```python
from build123d import *

# Parameters (mm, degrees)
SKETCH2_W               = 90
SKETCH2_H               = 45
BOSS_EXTRUDE1_DEPTH     = 8
SKETCH3_R               = 3.25
CUT_EXTRUDE1_DEPTH      = 10
SKETCH5_R               = 5.5
CUT_EXTRUDE2_DEPTH      = 5
SKETCH6_W               = 90
SKETCH6_H               = 5
BOSS_EXTRUDE2_DEPTH     = 32.5
SKETCH7_W               = 90
SKETCH7_H               = 3
BOSS_EXTRUDE3_DEPTH     = 45
SKETCH8_R               = 13
CUT_EXTRUDE4_DEPTH      = 13
BOSS_EXTRUDE6_START     = 5
SKETCH11_R              = 15
SKETCH11_R_2            = 13
BOSS_EXTRUDE6_DEPTH     = 5
FILLET1_R               = 2
CUT_EXTRUDE5_START      = -2
SKETCH12_R              = 13
CUT_EXTRUDE5_DEPTH      = 2
CUT_EXTRUDE6_DEPTH      = 67.494360663
CUT_EXTRUDE6_DEPTH_BACK = 67.494360663
SKETCH13_R              = 3
SKETCH14_R              = 9
CUT_EXTRUDE7_DEPTH      = 12
SKETCH16_W              = 90
SKETCH16_H              = 8
BOSS_EXTRUDE7_DEPTH     = 5
FILLET2_R               = 5


with BuildPart() as part:
    # Sketch2 → Boss-Extrude1 (new body)
    with BuildSketch(Plane(origin=(0, 0, 0), x_dir=(1, 0, 0), z_dir=(0, 1, 0))):
        Rectangle(SKETCH2_W, SKETCH2_H)
    extrude(amount=BOSS_EXTRUDE1_DEPTH)

    # Sketch3 → Cut-Extrude1 (cut)
    with BuildSketch(Plane(origin=(0, 8, 0), x_dir=(1, 0, 0), z_dir=(0, 1, 0))):
        with Locations(Location((12.5, 0, 0), (0, 0, 270))):
            Circle(SKETCH3_R)
        with Locations(Location((-12.5, 0, 0), (0, 0, 270))):
            Circle(SKETCH3_R)
    extrude(amount=-CUT_EXTRUDE1_DEPTH, mode=Mode.SUBTRACT)

    # Sketch5 → Cut-Extrude2 (cut)
    with BuildSketch(Plane(origin=(0, 8, 0), x_dir=(1, 0, 0), z_dir=(0, 1, 0))):
        with Locations(Location((-12.5, 0, 0), (0, 0, 270))):
            Circle(SKETCH5_R)
        with Locations(Location((12.5, 0, 0), (0, 0, 270))):
            Circle(SKETCH5_R)
    extrude(amount=-CUT_EXTRUDE2_DEPTH, mode=Mode.SUBTRACT)

    # Sketch6 → Boss-Extrude2 (add)
    with BuildSketch(Plane(origin=(0, 8, 0), x_dir=(1, 0, 0), z_dir=(0, 1, 0))):
        with Locations((0, -20)):
            Rectangle(SKETCH6_W, SKETCH6_H)
    extrude(amount=BOSS_EXTRUDE2_DEPTH)

    # Sketch7 → Boss-Extrude3 (add)
    with BuildSketch(Plane(origin=(0, 0, 17.5), x_dir=(-1, 0, 0), z_dir=(0, 0, -1))):
        with Locations((0, 39)):
            Rectangle(SKETCH7_W, SKETCH7_H)
    extrude(amount=BOSS_EXTRUDE3_DEPTH)

    # Sketch8 → Cut-Extrude4 (cut)
    with BuildSketch(Plane.XY.offset(22.5)):
        with Locations((0.439882225, 22.012295082)):
            Circle(SKETCH8_R)
    extrude(amount=-CUT_EXTRUDE4_DEPTH, mode=Mode.SUBTRACT)

    # Sketch11 → Boss-Extrude6 (add)
    with BuildSketch(Plane.XY.offset(22.5).offset(BOSS_EXTRUDE6_START)):
        with Locations(Location((0.439882225, 22.012295082, 0), (0, 0, 180))):
            Circle(SKETCH11_R)
        with Locations((0.439882225, 22.012295082)):
            Circle(SKETCH11_R_2, mode=Mode.SUBTRACT)
    extrude(amount=-BOSS_EXTRUDE6_DEPTH)

    # Fillet1
    fillet1_edges = [part.edges().sort_by_distance(p)[0] for p in [
        (15.439882225, 22.012295082, 22.5),
    ]]
    fillet(fillet1_edges, radius=FILLET1_R)

    # Sketch12 → Cut-Extrude5 (cut)
    with BuildSketch(Plane(origin=(0, 0, 17.5), x_dir=(-1, 0, 0), z_dir=(0, 0, -1)).offset(CUT_EXTRUDE5_START)):
        with BuildLine():
            Line((-28.100883588, 8), (27.221119137, 8))
            ThreePointArc((27.221119137, 8), (30.795754245, 22.781960072), (26.966438327, 37.5))
            Line((26.966438327, 37.5), (-27.846202777, 37.5))
            ThreePointArc((-27.846202777, 37.5), (-31.675518695, 22.781960072), (-28.100883588, 8))
        make_face()
        with Locations(Location((-0.439882225, 22.012295082, 0), (0, 0, 180))):
            Circle(SKETCH12_R, mode=Mode.SUBTRACT)
    extrude(amount=CUT_EXTRUDE5_DEPTH, mode=Mode.SUBTRACT)

    # Sketch13 → Cut-Extrude6 (cut, two sides: drawn at the far end of the back side and taken through both)
    with BuildSketch(Plane(origin=(0, 40.5, 0), x_dir=(1, 0, 0), z_dir=(0, 1, 0)).offset(-CUT_EXTRUDE6_DEPTH_BACK)):
        with Locations(Location((-30, 17.5, 0), (0, 0, 270))):
            Circle(SKETCH13_R)
        with Locations(Location((-10, 17.5, 0), (0, 0, 270))):
            Circle(SKETCH13_R)
        with Locations(Location((10, 17.5, 0), (0, 0, 270))):
            Circle(SKETCH13_R)
        with Locations(Location((30, 17.5, 0), (0, 0, 270))):
            Circle(SKETCH13_R)
    extrude(amount=CUT_EXTRUDE6_DEPTH + CUT_EXTRUDE6_DEPTH_BACK, mode=Mode.SUBTRACT)

    # Sketch14 → Cut-Extrude7 (cut)
    with BuildSketch(Plane(origin=(0, 40.5, 0), x_dir=(1, 0, 0), z_dir=(0, 1, 0))):
        with Locations(Location((-12.5, 0, 0), (0, 0, 270))):
            Circle(SKETCH14_R)
        with Locations(Location((12.5, 0, 0), (0, 0, 270))):
            Circle(SKETCH14_R)
    extrude(amount=-CUT_EXTRUDE7_DEPTH, mode=Mode.SUBTRACT)

    # Sketch16 → Boss-Extrude7 (add)
    with BuildSketch(Plane(origin=(0, 0, -22.5), x_dir=(-1, 0, 0), z_dir=(0, 0, -1))):
        with Locations((0, 4)):
            Rectangle(SKETCH16_W, SKETCH16_H)
    extrude(amount=BOSS_EXTRUDE7_DEPTH)

    # Fillet2
    fillet2_edges = [part.edges().sort_by_distance(p)[0] for p in [
        (36.550441794, 8, 17.5),
        (36.423101389, 37.5, 17.5),
        (-35.983219164, 37.5, 17.5),
        (-36.110559569, 8, 17.5),
    ]]
    fillet(fillet2_edges, radius=FILLET2_R)


solid = part.part
```
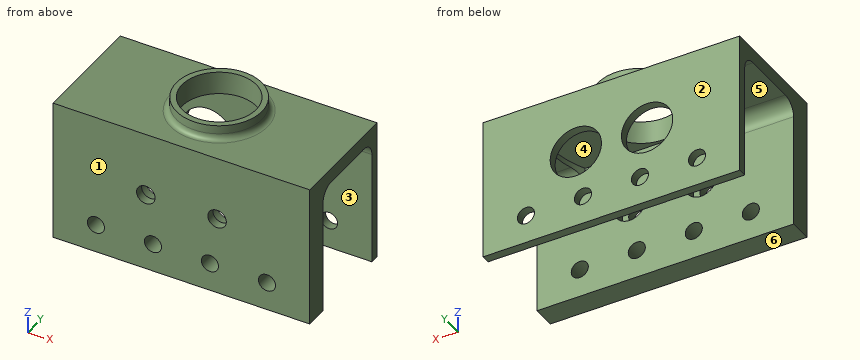
Read the model definition and answer for the solid it produces. Units are mm, in the model's axes. Face numbers are marked on the shaded views. A direction names the side the tool comes from. Coordinates: 2 decimals unless noted, no trailing zeros. Write each loop counter-clockwise with the first axis right and the second up, starting at its lowest first coordinate (ties: lowest second). Pieces come first, ordered by that corner, then holes. Notation, with made-up numbers: (-20.5, 65.5) -> (-1.5, 65.5) arc R11 ccw to (-1.5, 77.5) -> close; hole circle Ø1 at (52.25, -39.5). An arc over 180 degrees is marked (long way). Answer as a JSON object with one key per item and string values.
Q1. The part is cut by section C-C on x = 36. Give the vertices of the cut face in (y, z), then the cut area to 3 significant figures.
The answers:
{"outline": "(0, -27.5) -> (8, -27.5) -> (8, 12.5) arc R5 cw to (13, 17.5) -> (32.5, 17.5) arc R5 cw to (37.5, 12.5) -> (37.5, -27.5) -> (40.5, -27.5) -> (40.5, 22.5) -> (0, 22.5) -> close", "area": "708 mm2"}
Q2. The part is cut by section A-A on z = -22. Give the vertices of the cut face in (x, y), then the cut area to 3 significant figures.
The answers:
{"outline": "(-45, 0) -> (45, 0) -> (45, 8) -> (-45, 8) -> close; (-45, 37.5) -> (45, 37.5) -> (45, 40.5) -> (-45, 40.5) -> close", "area": "990 mm2"}
Q3. Consider line 1 (X direction, y = 38.1, z = -17.5); line 2 (X direction, y = 1.55, z = 0); line 3 (Y direction, x = -26.5, z = -6). Determine where each line is inside the solid, lowest interval first. Write a range as [from, to].
The answers:
{"line 1": "x = [-45, -33], [-27, -13], [-7, 7], [13, 27], [33, 45]", "line 2": "x = [-45, -15.75], [-9.25, 9.25], [15.75, 45]", "line 3": "y = [0, 8], [37.5, 40.5]"}
Q4. Determine the mould class of the marked faces 1, 2 and 3 for opening direction Y: pulls with the +Y half, pulls with the -Y half, needs draft (parallel to the pull), parting line crosses it, or undercut.
The answers:
{"face 1": "pulls with the -Y half", "face 2": "pulls with the +Y half", "face 3": "undercut"}
Q5. The part is cut by section B-B on z = 0. Give the number of separate pieces and of enclosed holes in the cut face, then the cut area to 3 significant figures.
The answers:
{"separate pieces": "6", "enclosed holes": "0", "area": "733 mm2"}
Q6. Flat-ended cylindrical pins translate along their axes: pin 1 Ø12 at (x, z) = (-12.5, -1.5) entering from +Y; pin 2 Ø17.5 at (x, y) = (-34.5, 25) entering from -Z; pin 3 Ø8 at (x, y) = (29, 22.5) entering from +Z. Find the tip coordinate at first contact, or state that the pin passes through.
The answers:
{"pin 1": "stops at y = 8", "pin 2": "stops at z = 17.34", "pin 3": "stops at z = 22.5"}
Q7. The part is cut by section D-D on z = 13.5. Give the vertices of the cut face in (x, y).
The answers:
{"outline": "(-45, 0) -> (45, 0) -> (45, 8.1) -> (28.15, 8.1) arc R31.24 cw to (28.1, 8) -> (-27.22, 8) arc R31.24 cw to (-27.27, 8.1) -> (-45, 8.1) -> close; (-45, 37.4) -> (-27.02, 37.4) arc R31.24 cw to (-26.97, 37.5) -> (27.85, 37.5) arc R31.24 cw to (27.9, 37.4) -> (45, 37.4) -> (45, 40.5) -> (-45, 40.5) -> close"}
Q8. A tool of negligible diameter and unlimited length cuts with its end or side. For the marked faces 4, 5 and 6, from which of +Z, -Z, +X, -X, +Y, -Y can it reach the whole face along a straight path? Write none if from no direction.
The answers:
{"face 4": "-Z", "face 5": "-Z, +X, -X", "face 6": "-Z, +X, -X, +Y, -Y"}
